```python
from build123d import *

# Parameters (mm, degrees)
BOSS_EXTRUDE1_DEPTH = 12.7
SKETCH2_R           = 1.778
CUT_EXTRUDE1_DEPTH  = 106.13339417
FILLET1_R           = 1.016


with BuildPart() as part:
    # Sketch1 → Boss-Extrude1 (new body)
    with BuildSketch(Plane.XY):
        with BuildLine():
            Line((-25.4, 0), (25.4, 0))
            ThreePointArc((25.4, 0), (31.75, -1.701477372), (36.398522628, -6.35))
            Line((36.398522628, -6.35), (61.798522628, -50.344090512))
            ThreePointArc((61.798522628, -50.344090512), (63.369186559, -54.875973564), (63.147095217, -59.6671764))
            Line((63.147095217, -59.6671764), (52.706203541, -82.822041569))
            Line((52.706203541, -82.822041569), (57.116867254, -57.807924643))
            ThreePointArc((57.116867254, -57.807924643), (57.116867254, -55.580256382), (56.354959836, -53.486932956))
            Line((56.354959836, -53.486932956), (30.954959836, -9.492842444))
            ThreePointArc((30.954959836, -9.492842444), (28.607157556, -7.145040164), (25.4, -6.285684887))
            Line((25.4, -6.285684887), (-25.4, -6.285684887))
            ThreePointArc((-25.4, -6.285684887), (-28.542842444, -3.142842444), (-25.4, 0))
        make_face()
    extrude(amount=BOSS_EXTRUDE1_DEPTH)

    # Sketch2 → Cut-Extrude1 (cut, through all)
    with BuildSketch(Plane.XY.offset(12.7)):
        with Locations((-25.4, -3.142842444)):
            Circle(SKETCH2_R)
    cut_extrude1 = extrude(amount=-CUT_EXTRUDE1_DEPTH, mode=Mode.SUBTRACT)

    # Mirror1: Cut-Extrude1 across plane
    add(cut_extrude1.mirror(Plane(origin=(0, 0, 0), x_dir=(0, 0, 1), z_dir=(1, 0, 0))), mode=Mode.SUBTRACT)

    # Fillet1
    fillet1_edges = [part.edges().sort_by_distance(p)[0] for p in [
        (52.706203541, -82.822041569, 6.35),
    ]]
    fillet(fillet1_edges, radius=FILLET1_R)


solid = part.part
```
Could you check a few things on this model? Use its own coordinates, in mm. A direction names the side the tool comes from. Coordinates: 2 decimals unless noted, no trailing zeros. Write each loop counter-clockwise with the first axis right and the second up, starting at its lowest first coordinate (ties: lowest second). Pieces come first, ordered by that corner, then holes. Notation, with made-up numbers: (-3.5, 87.25) -> (14.5, 87.25) arc R11 ccw to (14.5, 102.25) -> close; hole circle Ø10 at (-12.75, 67.25). An arc over 180 degrees is marked (long way). Write item = value, one per line. Start each with the question number.
(1) We'd pull the mould along X, two halves only. Please class faces 4 (the face through (0, 0, 6)), 5 (the face through (28.65, -7.17, 6.26)), 6 (the face through (27.176, -3.065, 6.439)), 7 (the face through (-27.176, -3.065, 6.439)): released by +X, released by -X, zero draft, split by the parting line, or undercut.
(2) Which directions (+Z, -Z, +X, -X, +Y, -Y) give clear straight access to the entire face, cutting with the end or side of a thin tool? Please do faces 1 (the face through (55.6, -66.4, 6.3)), 2 (the face through (0, -6.286, 6)), 3 (the face through (59.644, -67.435, 6.261)).
(3) I want a section at C-C (y = -63). Please give me the cut outline in (x, z).
(4) Will these pins go through, and if not, where does the flat tip stop? pin 1 (3 mm diameter, centred on y = -25, z = 3.5, fed in from +X); pin 2 (5 mm diameter, centred on x = 32, z = 1.5, fed in from -Y); pin 3 (5 mm diameter, centred on y = -28, z = 9.5, fed in from -X).
(5) I want a section at A-A (z = 4.75). Please give me the cut outline in (x, y), plus the area to 3 significant figures.
(6) I want a section at B-B (x = -20.5). Please give me the cut outline in (y, z).
(7) I need wall thicknesses on line 1 (Y direction, x = -25.4, z = 4.25); line 2 (Y direction, x = 21.5, z = 4.25); line 3 (X direction, y = -57, z = 3.75). Which ranges of each line are inside material? Lowest first, please. Write a range as [from, to].
Result set:
q1.face_4 = zero draft
q1.face_5 = released by -X
q1.face_6 = undercut
q1.face_7 = undercut
q2.face_1 = +Z, -Z, -X
q2.face_2 = +Z, -Z, -X, -Y
q2.face_3 = +Z, -Z, +X, -Y
q3.outline = (56.2, 0) -> (61.64, 0) -> (61.64, 12.7) -> (56.2, 12.7) -> close
q4.pin_1 = 48.03
q4.pin_2 = -15.63
q4.pin_3 = 40.2
q5.outline = (-25.4, -6.29) -> (25.4, -6.29) arc R6.41 cw to (30.95, -9.49) -> (56.35, -53.49) arc R6.41 cw to (57.12, -57.81) -> (54.12, -74.83) arc R1.02 ccw to (56.04, -75.42) -> (63.15, -59.67) arc R12.7 ccw to (61.8, -50.34) -> (36.4, -6.35) arc R12.7 ccw to (25.4, 0) -> (-25.4, 0) arc R3.14 ccw to start; hole circle Ø3.56 at (-25.4, -3.14); hole circle Ø3.56 at (25.4, -3.14)
q5.area = 814 mm2
q6.outline = (-6.29, 0) -> (0, 0) -> (0, 12.7) -> (-6.29, 12.7) -> close
q7.line_1 = [-6.29, -4.92], [-1.36, 0]
q7.line_2 = [-6.29, 0]
q7.line_3 = [57.21, 63.5]
